Autodesk Inventor part; units mm, degrees
ref_plane "YZ Plane" through (0, 0, 0) normal (1, 0, 0) x (0, 1, 0)
ref_plane "XZ Plane" through (0, 0, 0) normal (0, 1, 0) x (-1, 0, 0)
ref_plane "XY Plane" through (0, 0, 0) normal (0, 0, 1) x (1, 0, 0)
sketch "Esboço1" plane through (0, 0, 0) normal (0, 1, 0) x (-1, 0, 0)
  line L0 (-56.1514, 755.3759) -> (-111.1514, 755.3759)
  line L1 (-111.1514, 755.3759) -> (-111.1514, -847.6241)
  line L2 (-111.1514, -847.6241) -> (-56.1514, -847.6241)
  line L3 (-56.1514, -847.6241) -> (-56.1514, 755.3759)
  point P0 (0, 0)
  dimension "d0" = 1603
  dimension "d1" = 55
extrude "Extrusão1" add sketch "Esboço1" along normal blind 3
sketch "Esboço2" plane through (56.1514, 0, 755.3759) normal (0, 0, 1) x (1, 0, 0)
  circle A0 centre (28.1143, 53) radius 12.5
  circle A1 centre (28.1143, 53) radius 11
  line L0 (55, 3) -> (0, 3)
  line L1 (0, 3) -> (15.6143, 53)
  line L2 (40.6143, 53) -> (55, 3)
  point P0 (-56.1514, 0)
  point P1 (17.1143, 53)
  point P2 (39.1143, 53)
  dimension "d4" = 25
  dimension "d5" = 22
  dimension "d8" = 50
extrude "Extrusão2" add sketch "Esboço2" against normal blind 3 contours L2 L0 L1 A0
sketch "Esboço4" plane through (111.1514, 0, -847.6241) normal (0, 0, -1) x (-1, 0, 0)
  arc A0 (39.3857, 53) -> (14.3857, 53) centre (26.8857, 53) ccw
  line L0 (0, 3) -> (55, 3)
  circle A1 centre (26.8857, 53) radius 11
  circle A2 centre (26.8857, 53) radius 12.5
  line L1 (14.3857, 53) -> (0, 3)
  line L2 (55, 3) -> (39.3857, 53)
  point P0 (111.1514, 0)
  dimension "d40" = 22
extrude "Extrusão3" add sketch "Esboço4" against normal blind 3
sketch "Esboço5" plane through (0, 3, 0) normal (0, 1, 0) x (1, 0, 0)
  line L0 (56.1514, -749.3759) -> (95.2658, -749.3759)
  line L1 (111.1514, 844.6241) -> (56.1514, 844.6241)
  line L2 (56.1514, 847.6241) -> (56.1514, -755.3759)
  circle A0 centre (-124.6549, -214.6876) radius 2
  circle A1 centre (-96.9649, -152.5807) radius 2
  line L3 (16.1057, 85.4763) -> (84.2658, 124.8286)
  line L4 (84.2658, 124.8286) -> (152.4258, 85.4763)
  line L5 (152.4258, 85.4763) -> (152.4258, 6.7718)
  line L6 (152.4258, 6.7718) -> (84.2658, -32.5804)
  line L7 (84.2658, -32.5804) -> (16.1057, 6.7718)
  line L8 (16.1057, 6.7718) -> (16.1057, 85.4763)
  line L9 (56.1514, 847.6241) -> (56.1514, -755.3759)
  line L10 (111.1514, -755.3759) -> (111.1514, 847.6241)
  line L11 (56.1514, -755.3759) -> (111.1514, -755.3759)
  line L12 (111.1514, -755.3759) -> (111.1514, 847.6241)
  line L13 (111.1514, 847.6241) -> (56.1514, 847.6241)
  line L14 (56.1514, 847.6241) -> (56.1514, -755.3759)
  line L15 (95.2658, -755.3759) -> (95.2658, -755.3759)
  line L16 (90.2658, 847.6241) -> (78.2658, 847.6241)
  line L17 (95.2658, -752.3759) -> (95.2658, -752.3759)
  point P0 (111.1514, 841.6241)
  point P1 (56.1514, 841.6241)
  point P2 (84.2658, 46.1241)
  point P3 (73.2658, -755.3759)
  point P4 (73.2658, -755.3759)
  point P5 (84.2658, -755.3759)
  point P6 (84.2658, 847.6241)
  point P7 (84.2658, 847.6241)
  point P8 (73.2658, -752.3759)
  point P9 (84.2658, -752.3759)
  point P10 (111.1514, 109.3061)
  point P11 (111.1514, -17.058)
  point P12 (56.1514, -16.3486)
  point P13 (56.1514, 108.5967)
  dimension "d13" = 4
  dimension "d14" = 4
  dimension "d15" = 68
  dimension "d20" = 722.7955
  dimension "d22" = 722.7955
  dimension "d25" = 0
extrude "Extrusão4" add sketch "Esboço5" against normal blind 3 contours L4 L5 L6 L10 | L2 L7 L8 L3
sketch "Esboço6" plane through (0, 3, 0) normal (0, 1, 0) x (1, 0, 0)
  circle A0 centre (116.2657, 46.1244) radius 1.5
  circle A1 centre (52.2657, 46.1244) radius 1.5
  line L0 (16.1057, 85.4763) -> (16.1057, 6.7718)
  line L1 (152.4258, 6.7718) -> (152.4258, 85.4763)
  circle A2 centre (81.9973, 14.1244) radius 1.5
  circle A3 centre (81.9973, 78.1244) radius 1.5
  point P0 (0, 0)
  point P1 (56.1514, -16.3486)
  point P2 (56.1514, 108.5967)
  dimension "d28" = 3
  dimension "d29" = 3
  dimension "d30" = 64
  dimension "d31" = 36.16
  dimension "d43" = 3
  dimension "d44" = 3
  dimension "d45" = 64
  dimension "d46" = 32
  dimension "d47" = 32
  dimension "d48" = 36.1602
  dimension "d49" = 62.473
hole "Furo1" at (52.2657, 3, -46.1244) at (116.2657, 3, -46.1244) at (81.9973, 3, -14.1244) at (81.9973, 3, -78.1244) direction (0, -1, 0) diameter 3 depth 20 tip angle 118
extrude "Extrusão5" add sketch "Esboço2" against normal blind 3 contours A0
properties part number "Suporte Central Atualizado"
Geometry check sheet. Reference: the model listing, model coordinates, mm. A direction names the side the tool comes from. Round coordinates to 2 decimals unless told otherwise and drop trailing zeros. Loops run counter-clockwise (first coordinate to the right, second up) from the corner with the lowest first, then second, coordinate; pieces in that order, holes last. Notation, with made-up numbers: (4, 89.5) - (61, 89.5) arc R16 cw to (61, 97.5) - close; hole circle Ø6 at (81, 73). An arc over 180 degrees is marked (long way). Answer as CSV lines item,"result".
(1) Depth check by flat-ended pin: pin 1 Ø5 at (x, z) = (82, -14.12) entering from +Y; pin 2 Ø0.9 at (y, z) = (2, -359) entering from +X; pin 3 Ø1.5 at (y, z) = (1.5, -567) entering from -X. Enter the tip coordinate at first touch or a pass-through.
Output values:
pin 1,"stops at y = 3"
pin 2,"stops at x = 111.15"
pin 3,"stops at x = 56.15"
(2) Release check for a two-part mould opening along Z. For faces 3 (the face through (85, 0, -35)), 4 (the face through (83, 28, 752.376)), 5 (the face through (85, 3, -35)), 6 (the face through (83, 26, 755.376)) record: released by +Z, released by -Z, zero draft, split by the parting line, or undercut.
Output values:
face 3,"zero draft"
face 4,"undercut"
face 5,"undercut"
face 6,"released by +Z"
(3) Set-up check for faces 1 (the face through (84, 18, -847.624)), 2 (the face through (84, 28, -844.624)): record each of +Z, -Z, +X, -X, +Y, -Y from which the full face is reachable in a straight line by a thin tool's end or side.
Output values:
face 1,"-Z, +X, -X, +Y, -Y"
face 2,"+X, -X, +Y"
(4) Material ranges on line 1 along Z through (x, y) = (104.5, 14); line 2 along Y through (x, z) = (105.5, -343), recorded low to high.
Output values:
line 1,"z = -847.62 to -844.62, 752.38 to 755.38"
line 2,"y = 0 to 3"
(5) Cross-section at A-A, the plane y = 19. Enter the section's corners in (x, z), and give its area (3 significant figures).
Output values:
outline,"(61.15, -847.62) - (106.55, -847.62) - (106.55, -844.62) - (61.15, -844.62) - close; (61.15, 752.38) - (106.55, 752.38) - (106.55, 755.38) - (61.15, 755.38) - close"
area,"272 mm²"
(6) Cross-section at B-B, the plane z = 413. Enter the section's corners in (x, y).
Output values:
outline,"(56.15, 0) - (111.15, 0) - (111.15, 3) - (56.15, 3) - close"
